```python
from build123d import *

# Parameters (mm, degrees)
RESSALTO_EXTRUS_O1_DEPTH = 18
ESBO_O2_R                = 4
RESSALTO_EXTRUS_O2_DEPTH = 35
CHANFRO1_SIZE            = 1
PADR_OCIRCULAR1_COUNT    = 3
ESBO_O6_R                = 6
CORTE_EXTRUS_O1_DEPTH    = 3
ESBO_O6_4_R              = 4
CORTE_EXTRUS_O2_DEPTH    = 14


with BuildPart() as part:
    # Esbo_o1 → Ressalto-extrus_o1 (new body)
    with BuildSketch(Plane.XY):
        with BuildLine():
            ThreePointArc((-7, -12.124355653), (-2.064571939, -10.804514922), (2.03650339, -13.851088547))
            ThreePointArc((2.03650339, -13.851088547), (10.595070728, -9.15120081), (14, 0))
            ThreePointArc((14, 0), (10.389270368, 3.614285714), (10.977142857, 8.689207944))
            ThreePointArc((10.977142857, 8.689207944), (2.627637013, 13.75120081), (-7, 12.124355653))
            ThreePointArc((-7, 12.124355653), (-8.324698429, 7.190229208), (-13.013646247, 5.161880603))
            ThreePointArc((-13.013646247, 5.161880603), (-13.222707741, -4.6), (-7, -12.124355653))
        make_face()
    extrude(amount=RESSALTO_EXTRUS_O1_DEPTH)

    # Esbo_o2 → Ressalto-extrus_o2 (add)
    with BuildSketch(Plane.XY.offset(18)):
        Circle(ESBO_O2_R)
    extrude(amount=RESSALTO_EXTRUS_O2_DEPTH)

    # Chanfro1
    chanfro1_edges = [part.edges().sort_by_distance(p)[0] for p in [
        (-4, 0, 53),
    ]]
    chamfer(chanfro1_edges, length=CHANFRO1_SIZE)

    # Esbo_o5 → Rebaixo para SHCS M31 (revolve, cut)
    with BuildSketch(Plane(origin=(6.811116896, -5.882914807, 18), x_dir=(0, -1, 0), z_dir=(1, 0, 0))):
        Polygon((0, 0), (0, 18), (1.7, 18), (1.7, 3), (3.25, 3), (3.25, 0.125), (3.375, 0), align=None)
    rebaixo_para_shcs_m31 = revolve(axis=Axis((6.811116896, -5.882914807, 24.35), (0, 0, -1)), mode=Mode.SUBTRACT)

    # Padr_oCircular1: Rebaixo para SHCS M31 ×3 about axis
    padr_ocircular1_axis = Axis((0, 0, 0), (0, 0, 1))
    for i in range(1, PADR_OCIRCULAR1_COUNT):
        add(rebaixo_para_shcs_m31.rotate(padr_ocircular1_axis, i * 360 / PADR_OCIRCULAR1_COUNT), mode=Mode.SUBTRACT)

    # Esbo_o6 → Corte-extrus_o1 (cut)
    with BuildSketch(Plane(origin=(0, 0, 0), x_dir=(-1, 0, 0), z_dir=(0, 0, -1))):
        Circle(ESBO_O6_R)
    extrude(amount=-CORTE_EXTRUS_O1_DEPTH, mode=Mode.SUBTRACT)

    # Esbo_o6_4 → Corte-extrus_o2 (cut)
    with BuildSketch(Plane(origin=(0, 0, 0), x_dir=(-1, 0, 0), z_dir=(0, 0, -1))):
        with Locations(Location((0, 0, 0), (0, 0, 180))):
            Circle(ESBO_O6_4_R)
    extrude(amount=-CORTE_EXTRUS_O2_DEPTH, mode=Mode.SUBTRACT)


solid = part.part
```
Geometry: final body of the model. Coordinates: model frame, mm. A direction names the side the tool comes from. Coordinates: 2 decimals unless noted, no trailing zeros. Loops run counter-clockwise (first coordinate to the right, second up) from the corner with the lowest first, then second, coordinate; pieces in that order, holes last. Notation, with made-up numbers: (19, 37) -> (58, 37) arc R29 ccw to (58, 68) -> close; hole circle Ø9 at (7, -5.5). An arc over 180 degrees is marked (long way). Use a Markdown table: item, result. Add a question column.
(1) Section query D-D, the plane z = 28.5. Return loops of the section in (x, y).
(2) Section query A-A, the plane y = -11.5. Return loops of the section in (x, z).
(3) Line query: line 1 along Z through (x, y) = (-0.75, -0.25); line 2 along Y through (x, z) = (-9.75, 7); line 3 along Z through (x, y) = (-8, 4.75). Output: solid intervals per line, ascending.
(4) Mould query, pull axis X, two halves, no side actions, for faces 4 (the flat face through (-0.2, 9.4, 15)), 5 (the cylindrical face through (-0.867, -3.905, 34.762)), 6 (the cylindrical face through (-2.14, -10.79, 8.87)), 7 (the flat face through (0, 0, 53)). Classes: pulls with the +X half, pulls with the -X half, needs draft (parallel to the pull), parting line crosses it, or undercut.
(5) Pin query (flat end, axial travel): pin 1 Ø1.5 at (x, z) = (-6, 15) entering from -Y; pin 2 Ø10.5 at (x, y) = (-8.5, -2.96) entering from +Z; pin 3 Ø3 at (x, y) = (-8.5, -2.96) entering from +Z; pin 4 Ø6 at (x, y) = (-7, -7.5) entering from +Z. Return the tip coordinate at first contact, or that it passes through.
(6) Section query B-B, the plane z = 17. Return loops of the section in (x, y).
(7) Access query for faces 1 (the cylindrical face through (2.765, 13.724, 8.874)), 2 (the cylindrical face through (4.07, -7.63, 16.46)), 3 (the cylindrical face through (6, 0, 1)). Directions: +Z, -Z, +X, -X, +Y, -Y. A direction counts if a zero-diameter tool reaches every point of the face in a straight line with its end or side. Return the directions, or none.
(8) Section query C-C, the plane z = 5. Return loops of the section in (x, y).
Answer:
| question | item | result |
|---|---|---|
| 1 | outline | circle Ø8 at (0, 0) |
| 2 | outline | (-7.98, 0) -> (-6.12, 0) -> (-6.12, 18) -> (-7.98, 18) -> close; (-0.21, 0) -> (7.98, 0) -> (7.98, 18) -> (-0.21, 18) -> close |
| 3 | line 1 | z = 14 to 53 |
| 3 | line 2 | y = -10.05 to -4.11, -1.8 to 5.99 |
| 3 | line 3 | z = 0 to 18 |
| 4 | face 4 | undercut |
| 4 | face 5 | parting line crosses it |
| 4 | face 6 | undercut |
| 4 | face 7 | needs draft |
| 5 | pin 1 | stops at y = -11.92 |
| 5 | pin 2 | stops at z = 52.25 |
| 5 | pin 3 | passes through |
| 5 | pin 4 | stops at z = 18 |
| 6 | outline | (-13.01, 5.16) arc R14 ccw to (-7, -12.12) arc R5.87 cw to (2.04, -13.85) arc R14 ccw to (14, 0) arc R5.87 cw to (10.98, 8.69) arc R14 ccw to (-7, 12.12) arc R5.87 cw to start; hole circle Ø6.5 at (-8.5, -2.96); hole circle Ø6.5 at (1.69, 8.84); hole circle Ø6.5 at (6.81, -5.88) |
| 7 | face 1 | +Z, -Z, +Y |
| 7 | face 2 | +Z |
| 7 | face 3 | -Z |
| 8 | outline | (-13.01, 5.16) arc R14 ccw to (-7, -12.12) arc R5.87 cw to (2.04, -13.85) arc R14 ccw to (14, 0) arc R5.87 cw to (10.98, 8.69) arc R14 ccw to (-7, 12.12) arc R5.87 cw to start; hole circle Ø3.4 at (-8.5, -2.96); hole circle Ø8 at (0, 0); hole circle Ø3.4 at (1.69, 8.84); hole circle Ø3.4 at (6.81, -5.88) |
